Design review of the part built by this model. Coordinates are the model's own, in mm. A direction names the side the tool comes from. Round coordinates to 2 decimals unless told otherwise and drop trailing zeros. Loops run counter-clockwise (first coordinate to the right, second up) from the corner with the lowest first, then second, coordinate; pieces in that order, holes last. Notation, with made-up numbers: (-37, 22) - (21, 22) arc R23 cw to (21, 48) - close; hole circle Ø10 at (77, 53). An arc over 180 degrees is marked (long way). Return JSON: item names as keys, results as strings. Group by question number.
from build123d import *

# Parameters (mm, degrees)
SKETCH1_W           = 90
SKETCH1_H           = 45
BOSS_EXTRUDE1_DEPTH = 117
BOSS_EXTRUDE2_START = -72
BOSS_EXTRUDE2_DEPTH = 45
BOSS_EXTRUDE4_START = -90
SKETCH1_5_W         = 90
SKETCH1_5_H         = 9
BOSS_EXTRUDE4_DEPTH = 27
BOSS_EXTRUDE5_START = -90
BOSS_EXTRUDE5_DEPTH = 27
CUT_EXTRUDE1_DEPTH  = 173.884354411
RIB4_REACH          = 186.225
SKETCH5_WALL_W      = 421.362499074
SKETCH5_WALL_H      = 10


with BuildPart() as part:
    # Sketch1 → Boss-Extrude1 (new body)
    with BuildSketch(Plane.XY):
        with Locations((45, 22.5)):
            Rectangle(SKETCH1_W, SKETCH1_H)
    extrude(amount=-BOSS_EXTRUDE1_DEPTH)

    # Sketch1_3 → Boss-Extrude2 (add)
    with BuildSketch(Plane.XY.offset(BOSS_EXTRUDE2_START)):
        Polygon((0, 81), (0, 45), (68.497865987, 45), (90, 45), (90, 81), align=None)
    extrude(amount=-BOSS_EXTRUDE2_DEPTH)

    # Sketch1_5 → Boss-Extrude4 (add)
    with BuildSketch(Plane.XY.offset(BOSS_EXTRUDE4_START)):
        with Locations((45, 85.5)):
            Rectangle(SKETCH1_5_W, SKETCH1_5_H)
    extrude(amount=-BOSS_EXTRUDE4_DEPTH)

    # Sketch1_6 → Boss-Extrude5 (add)
    with BuildSketch(Plane.XY.offset(BOSS_EXTRUDE5_START)):
        with BuildLine():
            ThreePointArc((90, 90), (45, 135), (0, 90))
            Line((0, 90), (18, 90))
            ThreePointArc((18, 90), (45, 117), (72, 90))
            Line((72, 90), (90, 90))
        make_face()
    extrude(amount=-BOSS_EXTRUDE5_DEPTH)

    # Sketch2 → Cut-Extrude1 (cut, through all)
    with BuildSketch(Plane(origin=(0, 45, 0), x_dir=(1, 0, 0), z_dir=(0, 1, 0))):
        with BuildLine():
            Line((18, 0), (72, 0))
            ThreePointArc((72, 0), (45, 27), (18, 0))
        make_face()
    extrude(amount=-CUT_EXTRUDE1_DEPTH, mode=Mode.SUBTRACT)

    # Sketch5 wall → Rib4 (add, up to next)
    with BuildSketch(Plane(origin=(45, 63, -54), x_dir=(0, -0.707106781187, 0.707106781187), z_dir=(0, -0.707106781187, -0.707106781187)), mode=Mode.PRIVATE) as rib4_sk1:
        Rectangle(SKETCH5_WALL_W, SKETCH5_WALL_H)
    rib4_tool1 = extrude(rib4_sk1.sketch, amount=RIB4_REACH, mode=Mode.PRIVATE) - part.part
    add(rib4_tool1.solids().sort_by_distance((45, 63, -54))[0])


solid = part.part
Q1. Add section A-A, the plane x = 45. State the section outline as (y, z) points, plus the area to 3 significant figures.
Q2. Tool access review of faces 1 (the flat face through (40, 56, -61)), 2 (the flat face through (70, 63, -72)), 3 (the cylindrical face through (44.406, 116.993, -103.311)): name each direction out of +Z, -Z, +X, -X, +Y, -Y from which nothing blocks a thin tool from reaching the whole face with its end or side.
Q3. Add section C-C, the plane y = 28. State the section outline as (x, z) points.
Q4. Insertion check: pin 1 Ø4 at (y, z) = (110.5, -104.5) entering from -X; pin 2 Ø8 at (x, z) = (64, -39.5) entering from -Y; pin 3 Ø20 at (x, z) = (45, -77) entering from +Y; pin 4 Ø11 at (y, z) = (61, -46.5) entering from -X. Each pin has a flat end and moves straight along its axis. Give the tip position at first contact, or say it passes through.
Q5. Add section D-D, the plane z = -9.5. State the section outline as (x, y) points.
Q6. Add section B-B, the plane z = -62.5. State the section outline as (x, y) points.
Q7. For line 1 (Z direction, x = 15, y = 94); line 2 (Y direction, x = 36.5, z = -47.5); line 3 (Z direction, x = 17, y = 49.5), list the stretches that pass through material, from the lowest coordinate up.
Q8. Draft analysis for pull direction X (two halves, no side actions). For faces 4 (the flat face through (0, 34, -71)), 5 (the flat face through (90, 34, -71)), 6 (the flat face through (44, 0, -58)), 7 (the flat face through (45, 90, -103)), state which applies: pulls with the +X half, pulls with the -X half, needs draft (parallel to the pull), parting line crosses it, or undercut.
Evaluation:
{
 "1": {"outline": "(0, -117) - (90, -117) - (90, -90) - (81, -90) - (81, -72) - (45, -36) - (45, -27) - (0, -27) - close; (117, -117) - (135, -117) - (135, -90) - (117, -90) - close", "area": "7,050 mm²"},
 "2": {"face 1": "+Z, -X, +Y", "face 2": "+Z, +X, +Y", "face 3": "+Z, -Z"},
 "3": {"outline": "(0, -117) - (90, -117) - (90, 0) - (72, 0) arc R27 cw to (18, 0) - (0, 0) - close"},
 "4": {"pin 1": "x = 3.98", "pin 2": "y = 0", "pin 3": "y = 81", "pin 4": "x = 40"},
 "5": {"outline": "(0, 0) - (19.73, 0) - (19.73, 45) - (0, 45) - close; (70.27, 0) - (90, 0) - (90, 45) - (70.27, 45) - close"},
 "6": {"outline": "(0, 0) - (90, 0) - (90, 45) - (50, 45) - (50, 71.5) - (40, 71.5) - (40, 45) - (0, 45) - close"},
 "7": {"line 1": "-117 to -90", "line 2": "0 to 45", "line 3": "-117 to -72"},
 "8": {"face 4": "pulls with the -X half", "face 5": "pulls with the +X half", "face 6": "needs draft", "face 7": "undercut"}
}
